Can you work these out from the model? Positions are in its coordinate system, mm. Round coordinates to 2 decimals unless told otherwise and drop trailing zeros. Loops run counter-clockwise (first coordinate to the right, second up) from the corner with the lowest first, then second, coordinate; pieces in that order, holes last. Notation, with made-up numbers: (44.5, -24) -> (58.5, -24) arc R21 ccw to (58.5, 1) -> close; hole circle Ø5 at (78, 34.25). An arc over 180 degrees is marked (long way). Write each question's results on one line, items separated by ' | '.
from build123d import *

# Parameters (mm, degrees)
F0_W      = 15.89278
F0_H      = 118.7259927564
F1_DEPTH  = 5.08
F2_W      = 15.9494206481
F2_H      = 5.08
F3_DEPTH  = 25.4
F4_W      = 16.0588771277
F4_H      = 5.08
F5_DEPTH  = 25.4
F6_DEPTH  = 12.7
F7_DEPTH  = 25.4
F8_W      = 6.35
F8_H      = 12.7
F9_DEPTH  = 25.4
F10_DEPTH = 1.27


with BuildPart() as f1:
    # F0 (on Top) → F1 (new body)
    with BuildSketch(Plane.XY):
        with Locations((7.94639, 59.3629963782)):
            Rectangle(F0_W, F0_H)
    extrude(amount=F1_DEPTH)

    # F2 (on face) → F3 (join)
    with BuildSketch(Plane.YZ.offset(15.89278)):
        with Locations((110.7512824323, 2.54)):
            Rectangle(F2_W, F2_H)
    extrude(amount=F3_DEPTH)

    # F4 (on face) → F5 (join)
    with BuildSketch(Plane(origin=(0, 0, 0), x_dir=(0, -1, 0), z_dir=(-1, 0, 0))):
        with Locations((-110.6965541926, 2.54)):
            Rectangle(F4_W, F4_H)
    extrude(amount=F5_DEPTH)

    # F6 (add): a face of the model
    f6_faces = [f1.faces().sort_by_distance(p)[0] for p in [
        (7.94639, 118.7259927564, 2.54),
    ]]
    extrude(f6_faces, amount=F6_DEPTH)

    # F7 (add): a face of the model
    f7_faces = [f1.faces().sort_by_distance(p)[0] for p in [
        (7.94639, 0, 2.54),
    ]]
    extrude(f7_faces, amount=F7_DEPTH)

    # F8 (on face) → F9 (cut)
    with BuildSketch(Plane.XY.offset(5.08)):
        with Locations((7.94639, 118.5111179948)):
            Rectangle(F8_W, F8_H)
    extrude(amount=-F9_DEPTH, mode=Mode.SUBTRACT)

    # F10 (add): a face of the model
    f10_faces = [f1.faces().sort_by_distance(p)[0] for p in [
        (7.9315574243, 75.7859315554, 5.08),
    ]]
    extrude(f10_faces, amount=F10_DEPTH)


solid = f1.part
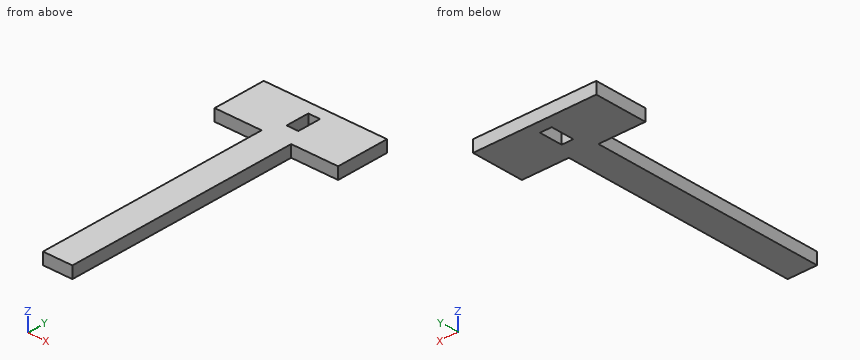
1. Please list where these lines run through material, in increasing order: line 1 (Y direction, x = 8, z = 5.5); line 2 (X direction, y = 67, z = 1); line 3 (Y direction, x = -17.5, z = 0.5). Write a range as from..to.
Final values:
line 1: -25.4..112.16, 124.86..131.43 | line 2: 0..15.89 | line 3: 102.67..131.43
2. If we section it at A-A (y = 116.5): List the corners of the cut face in (x, z) for me, then the cut area to 3 significant figures.
Final values:
outline: (-25.4, 0) -> (4.77, 0) -> (4.77, 6.35) -> (-25.4, 6.35) -> close; (11.12, 0) -> (41.29, 0) -> (41.29, 6.35) -> (11.12, 6.35) -> close | area: 383 mm2
3. If we section it at B-B (z = 1.5): List the corners of the cut face in (x, y) for me.
Final values:
outline: (-25.4, 102.67) -> (0, 102.67) -> (0, -25.4) -> (15.89, -25.4) -> (15.89, 102.78) -> (41.29, 102.78) -> (41.29, 131.43) -> (-25.4, 131.43) -> close; hole (4.77, 112.16) -> (11.12, 112.16) -> (11.12, 124.86) -> (4.77, 124.86) -> close
4. Will these pins go through, and if not, where does the flat tip stop? pin 1 (3 mm diameter, centred on x = 22.5, z = 2, fed in from -Y); pin 2 (3 mm diameter, centred on y = 20, z = 1.5, fed in from +X); pin 3 (1.9 mm diameter, centred on x = -7.5, z = 3, fed in from -Y).
Final values:
pin 1: y = 102.78 | pin 2: x = 15.89 | pin 3: y = 102.67
5. If we section it at C-C (y = 86): List the corners of the cut face in (x, z) for me.
Final values:
outline: (0, 0) -> (15.89, 0) -> (15.89, 6.35) -> (0, 6.35) -> close
6. If we section it at D-D (x = -10): List the corners of the cut face in (y, z) for me, then the cut area to 3 significant figures.
Final values:
outline: (102.67, 0) -> (131.43, 0) -> (131.43, 6.35) -> (102.67, 6.35) -> close | area: 183 mm2
